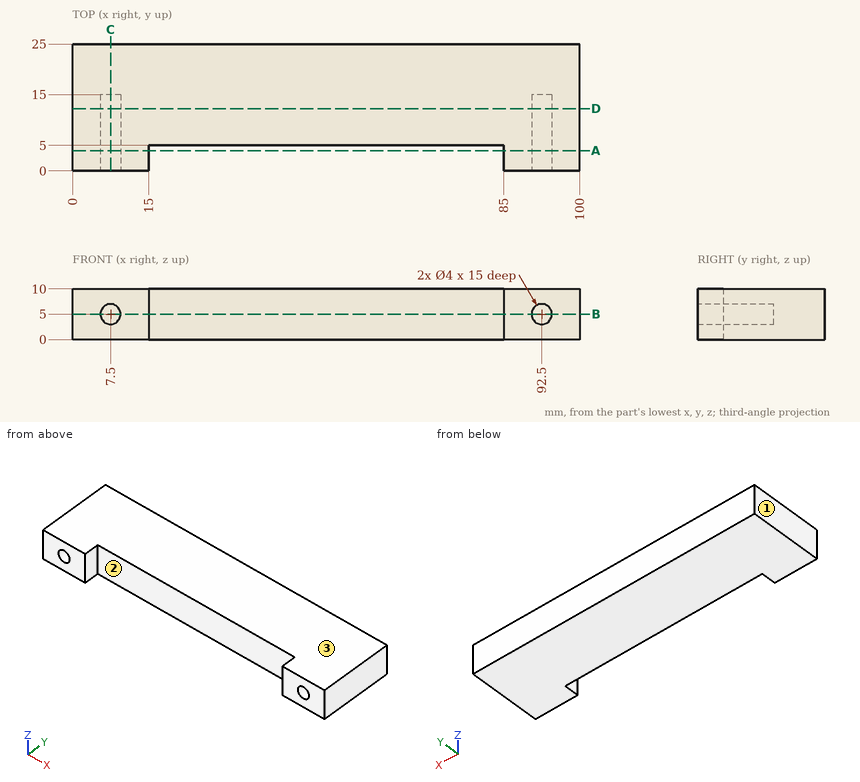
Can you work these out from the drawing? Everything is in mm from the part's minimum corner. Round coordinates to 2 decimals unless told otherwise and drop trailing zeros. Loops run counter-clockwise (first coordinate to the right, second up) from the corner with the lowest first, then second, coordinate; pieces in that order, holes last. Notation, with made-up numbers: (1.25, 47.5) -> (25.25, 47.5) arc R17 cw to (25.25, 67.5) -> close; hole circle Ø6 at (8.5, -23). An arc over 180 degrees is marked (long way). Use CSV: the item, a comma, the result in double quotes.
(1) If I drill on probe 1 along X at (y, z) = (8.75, 5); probe 2 along X at (y, z) = (4.75, 5); probe 3 along X at (y, z) = (1.25, 1.25), over which ranges is the centre line in solid material (lowest first)? Write a range as [from, to].
Return value:
probe 1,"x = [0, 5.5], [9.5, 90.5], [94.5, 100]"
probe 2,"x = [0, 5.5], [9.5, 15], [85, 90.5], [94.5, 100]"
probe 3,"x = [0, 15], [85, 100]"
(2) If we mould it in two halves opening along X, with no side actions, what happens to the marked faces 1, 2 and 3? For each: +X half, -X half, draft (parallel to the pull), parting line (faces both ways), or undercut.
Return value:
face 1,"-X half"
face 2,"undercut"
face 3,"draft"
(3) Suppose I cut it at A-A on y = 4. Write out the boundary of the cut face in (x, z), plus the area to 3 significant figures.
Return value:
outline,"(0, 0) -> (15, 0) -> (15, 10) -> (0, 10) -> close; (85, 0) -> (100, 0) -> (100, 10) -> (85, 10) -> close; hole circle Ø4 at (7.5, 5); hole circle Ø4 at (92.5, 5)"
area,"275 mm²"
(4) Will these pins go through, and if not, where does the flat tip stop? pin 1 Ø6 at (x, z) = (47, 4.5) entering from -Y; pin 2 Ø1 at (x, y) = (66, 5) entering from -Z.
Return value:
pin 1,"stops at y = 5"
pin 2,"stops at z = 0"
(5) Suppose I cut it at D-D on y = 12.25. Write out the boundary of the cut face in (x, z).
Return value:
outline,"(0, 0) -> (100, 0) -> (100, 10) -> (0, 10) -> close; hole circle Ø4 at (7.5, 5); hole circle Ø4 at (92.5, 5)"
(6) Suppose I cut it at C-C on x = 7.5. Write out the boundary of the cut face in (y, z).
Return value:
outline,"(0, 0) -> (25, 0) -> (25, 10) -> (0, 10) -> (0, 7) -> (15, 7) -> (15, 3) -> (0, 3) -> close"
(7) Suppose I cut it at B-B on z = 5. Write out the boundary of the cut face in (x, y).
Return value:
outline,"(0, 0) -> (5.5, 0) -> (5.5, 15) -> (9.5, 15) -> (9.5, 0) -> (15, 0) -> (15, 5) -> (85, 5) -> (85, 0) -> (90.5, 0) -> (90.5, 15) -> (94.5, 15) -> (94.5, 0) -> (100, 0) -> (100, 25) -> (0, 25) -> close"
